Source: CAD feature listing. Evaluate the final solid. Frame: model axes, mm. A direction names the side the tool comes from. Give positions to 0.01 mm unless a question says otherwise; leave off trailing zeros. Write each loop counter-clockwise with the first axis right and the second up, starting at its lowest first coordinate (ties: lowest second). Pieces come first, ordered by that corner, then holes. Notation, with made-up numbers: M -38,-4.5 L -30,-4.5 A10 cw -30,11.5 Z; hole C -14,32 d1. An arc over 180 degrees is marked long. Use CSV: the item, a comma, the result in double quotes. Start each with the question number.
from build123d import *

# Parameters (mm, degrees)
F0_W      = 52.4384081364
F0_H      = 12.3928444714
F1_DEPTH  = 5
F2_W      = 47.5675082519
F2_H      = 12.3928444714
F3_DEPTH  = 0.4
F4_W      = 17.4495708197
F4_H      = 2.7426069784
F5_DEPTH  = 0.6
F6_W      = 7.059096708
F6_H      = 2.7426069784
F7_DEPTH  = 1.4
F8_W      = 3.7224081942
F8_H      = 8.9364917949
F9_DEPTH  = 1.3
F10_W     = 1.8612040971
F10_H     = 8.6072823033
F11_DEPTH = 1.5


with BuildPart() as f1:
    # F0 (on Front) → F1 (new body)
    with BuildSketch(Plane.XZ):
        with Locations((3.5388600081, 16.1491944455)):
            Rectangle(F0_W, F0_H)
    extrude(amount=F1_DEPTH)

    # F2 (on face) → F3 (join)
    with BuildSketch(Plane.XZ.offset(5)):
        with Locations((5.9743099503, 16.1491944455)):
            Rectangle(F2_W, F2_H)
    extrude(amount=F3_DEPTH)

    # F4 (on face) → F5 (cut)
    with BuildSketch(Plane.XY.offset(22.3456166812)):
        with Locations((2.9753278941, -3.6286965108)):
            Rectangle(F4_W, F4_H)
    extrude(amount=-F5_DEPTH, mode=Mode.SUBTRACT)

    # F6 (on face) → F7 (join)
    with BuildSketch(Plane.XY.offset(21.7456166812)):
        with Locations((-2.2199091618, -3.6286965108)):
            Rectangle(F6_W, F6_H)
    extrude(amount=F7_DEPTH)

    # F8 (on face) → F9 (cut)
    with BuildSketch(Plane.YZ.offset(29.7580640763)):
        with Locations((-2.8406968922, 16.1491944455)):
            Rectangle(F8_W, F8_H)
    extrude(amount=-F9_DEPTH, mode=Mode.SUBTRACT)

    # F10 (on face) → F11 (join)
    with BuildSketch(Plane.YZ.offset(28.4580640763)):
        with Locations((-1.9100948437, 16.3137991913)):
            Rectangle(F10_W, F10_H)
    extrude(amount=F11_DEPTH)


solid = f1.part
Item 1: Section B-B (x = 5). Return the cut outline in (y, z), plus the area to 3 significant figures.
Item 2: Set-up query: faces 4 (the flat face through (6, -4, 21.746)), 5 (the flat face through (6, -5.4, 16)), 6 (the flat face through (29, -2.841, 16)). Return all of +Z, -Z, +X, -X, +Y, -Y with unobstructed straight access to the full face (end or side cutting, diameter ignored); none if empty.
Item 3: Section C-C (z = 15.5). Return the cut outline in (x, y), plus the area to 3 significant figures.
Item 4: Pull-direction query (Y, two-part tool) for faces 1 (the flat face through (29.758, -0.3, 16.1)), 2 (the flat face through (-20, -5, 16)), 3 (the flat face through (29, -2, 12.01)); classes: released by +Y, released by -Y, zero draft, split by the parting line, or undercut.
Item 5: Material intervals for probe 1 along Z at (x, y) = (-18, -2.35); probe 2 along X at (y, z) = (-3.3, 12.25); probe 3 along X at (y, z) = (-0.8, 21.25), sorted ascending.
Item 6: Section D-D (x = -12). Return the cut outline in (y, z).
Item 7: Section A-A (y = -1.6). Return the cut outline in (x, z), plus the area to 3 significant figures.
Item 8: Contact query for flat-ended pins moving along their axis: pin 1 Ø6 at (x, z) = (-5.5, 15) entering from +Y; pin 2 Ø0.7 at (y, z) = (-3, 22) entering from +X; pin 3 Ø0.6 at (x, z) = (-0.5, 23) entering from -Y; pin 4 Ø1 at (x, y) = (16.5, -4.5) entering from +Z. Output: stop coordinate, or through.
Output values:
1,outline,"M -5.4,9.95 L 0,9.95 L 0,22.35 L -2.26,22.35 L -2.26,21.75 L -5,21.75 L -5,22.35 L -5.4,22.35 Z"
1,area,"65.3 mm2"
2,face 4,"+Z"
2,face 5,"+Z, -Z, +X, -X, -Y"
2,face 6,"+X"
3,outline,"M -22.68,-5 L -17.81,-5 L -17.81,-5.4 L 29.76,-5.4 L 29.76,-4.7 L 28.46,-4.7 L 28.46,-2.84 L 29.96,-2.84 L 29.96,-0.98 L 29.76,-0.98 L 29.76,0 L -22.68,0 Z"
3,area,"279 mm2"
4,face 1,"zero draft"
4,face 2,"released by -Y"
4,face 3,"undercut"
5,probe 1,"z = 9.95 to 22.35"
5,probe 2,"x = -22.68 to 28.46"
5,probe 3,"x = -22.68 to 29.76"
6,outline,"M -5.4,9.95 L 0,9.95 L 0,22.35 L -5.4,22.35 Z"
7,outline,"M -22.68,9.95 L 29.76,9.95 L 29.76,11.68 L 28.46,11.68 L 28.46,12.01 L 29.96,12.01 L 29.96,20.62 L 29.76,20.62 L 29.76,22.35 L -22.68,22.35 Z"
7,area,"651 mm2"
8,pin 1,"stops at y = 0"
8,pin 2,"stops at x = 29.76"
8,pin 3,"stops at y = -5"
8,pin 4,"stops at z = 22.35"
